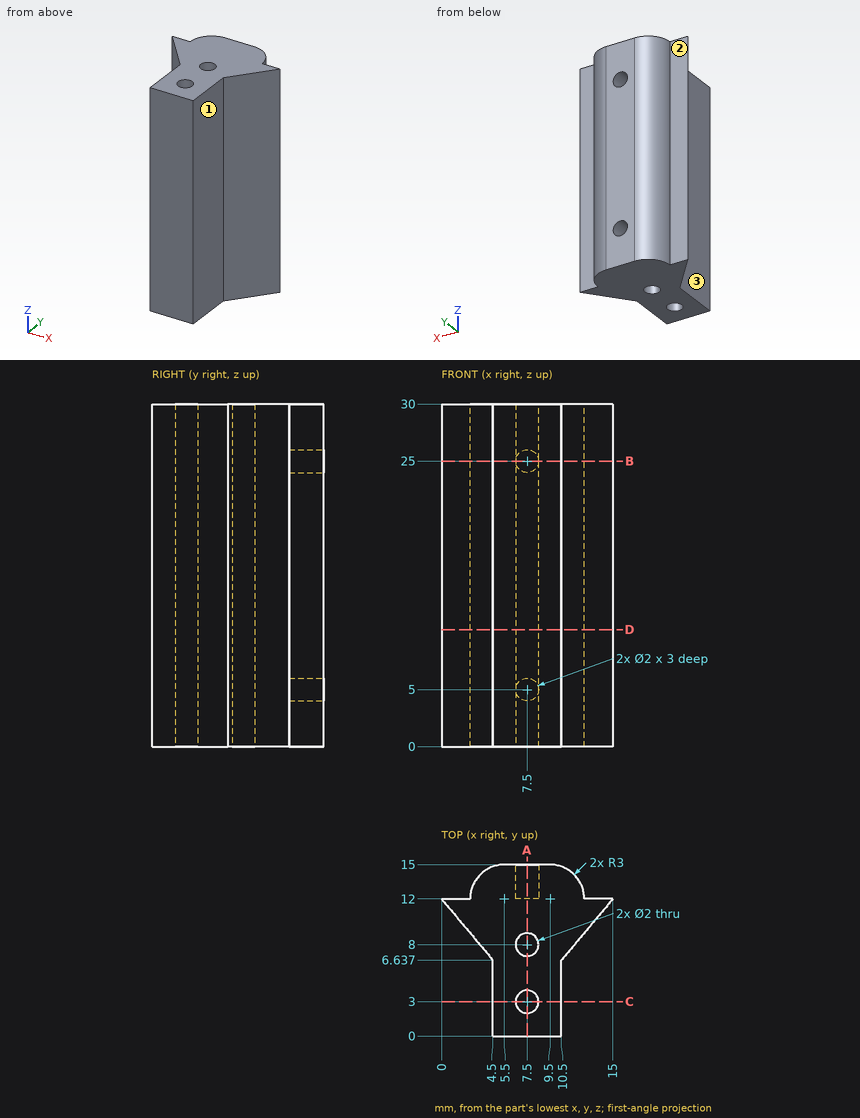
Part print with two shaded views. Sizes in mm from the minimum x, y, z corner. A direction names the side the tool comes from. Round coordinates to 2 decimals unless told otherwise and drop trailing zeros. Write each loop counter-clockwise with the first axis right and the second up, starting at its lowest first coordinate (ties: lowest second). Pieces come first, ordered by that corner, then holes. Notation, with made-up numbers: (-34.75, 44) -> (-12.75, 44) arc R21 ccw to (-12.75, 77) -> close; hole circle Ø8 at (71.5, -7.5). An arc over 180 degrees is marked (long way). Use one line per item in the form item = value.
Q1. Band-saw the part on D-D, the plane z = 10.25. Write the cut outline in (x, y).
Conclusion:
outline = (0, 12) -> (4.5, 6.64) -> (4.5, 0) -> (10.5, 0) -> (10.5, 6.64) -> (15, 12) -> (12.5, 12) arc R3 ccw to (9.5, 15) -> (5.5, 15) arc R3 ccw to (2.5, 12) -> close; hole circle Ø2 at (7.5, 3); hole circle Ø2 at (7.5, 8)
Q2. Drill centre lines: L1, parallel to Z at x = 7.5, y = 14.3; L2, parallel to Y at x = 7.5, z = 18.5; L3, parallel to X at y = 13.7, z = 5. Where is each one in solid material? Low to high.
Conclusion:
L1 = 0 to 4, 6 to 24, 26 to 30
L2 = 0 to 2, 4 to 7, 9 to 15
L3 = 3.03 to 6.5, 8.5 to 11.97
Q3. Band-saw the part on A-A, the plane x = 7.5. Write the cut outline in (y, z), then the cut area to 3 significant figures.
Conclusion:
outline = (0, 0) -> (2, 0) -> (2, 30) -> (0, 30) -> close; (4, 0) -> (7, 0) -> (7, 30) -> (4, 30) -> close; (9, 0) -> (15, 0) -> (15, 4) -> (12, 4) -> (12, 6) -> (15, 6) -> (15, 24) -> (12, 24) -> (12, 26) -> (15, 26) -> (15, 30) -> (9, 30) -> close
area = 318 mm²
Q4. Band-saw the part on B-B, the plane z = 25. Write the cut outline in (x, y).
Conclusion:
outline = (0, 12) -> (4.5, 6.64) -> (4.5, 0) -> (10.5, 0) -> (10.5, 6.64) -> (15, 12) -> (12.5, 12) arc R3 ccw to (9.5, 15) -> (8.5, 15) -> (8.5, 12) -> (6.5, 12) -> (6.5, 15) -> (5.5, 15) arc R3 ccw to (2.5, 12) -> close; hole circle Ø2 at (7.5, 3); hole circle Ø2 at (7.5, 8)
Q5. Tool access for the marked faces 1, 2 and 3: list every direction of +Z, -Z, +X, -X, +Y, -Y with a clear straight run to the whole face (end or side of a thin tool).
Conclusion:
face_1 = +Z, -Z, +X, -Y
face_2 = +Z, -Z, -X, +Y
face_3 = +Z, -Z, -X, -Y
Q6. Band-saw the part on C-C, the plane y = 3. Write the cut outline in (x, z).
Conclusion:
outline = (4.5, 0) -> (6.5, 0) -> (6.5, 30) -> (4.5, 30) -> close; (8.5, 0) -> (10.5, 0) -> (10.5, 30) -> (8.5, 30) -> close
Q7. Drop flat-ended pins along their axis: P1, Ø2, axis at x = 1, z = 11.5, coming from the +Y side; P2, Ø1.8, axis at x = 7.5, z = 5, coming from the -Y side; P3, Ø5.5, axis at y = 3, z = 14.5, coming from the -X side; P4, Ø3.5, axis at y = 2, z = 10, coming from the +X side. Give the stop position or say it passes through.
Conclusion:
P1 = 12
P2 = 0
P3 = 4.5
P4 = 10.5
